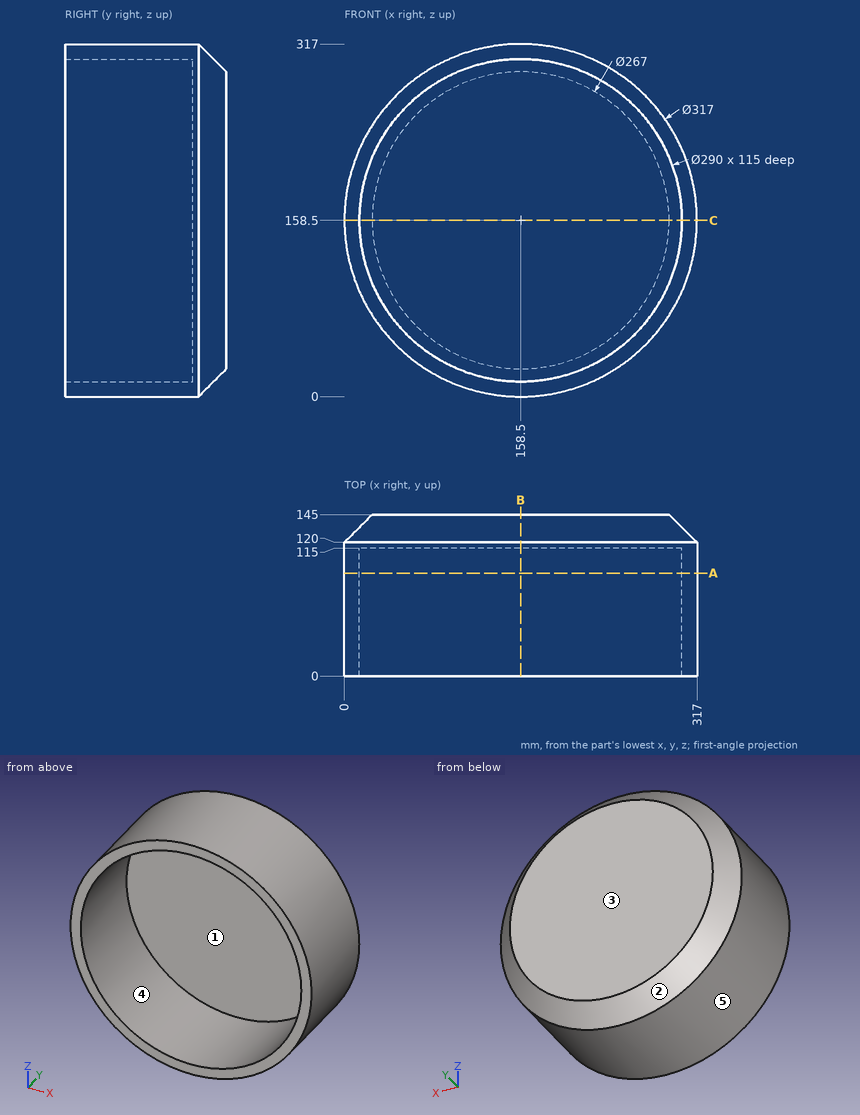
Here's the drawing with two shaded views (mm, measured from the low corner). I have some questions. A direction names the side the tool comes from. Coordinates: 2 decimals unless noted, no trailing zeros. Order: outer loops, then holes, each group sorted by start corner. A loop starts at its lowest first (then second) coordinate and runs counter-clockwise, first axis right, second up.
Q1. Thinking about a two-plate mould opening in X: for the marked faces 3, 4 and 5, which applies, released by +X, released by -X, zero draft, split by the parting line, or undercut?
Q2. Suppose I cut it at B-B on x = 158.5. Please give me the cut outline in (y, z), and give its area (3 significant figures).
Q3. Suppose I cut it at A-A on y = 92.5. Please give me the cut outline in (x, z), and give its area (3 significant figures).
Q4. Suppose I cut it at C-C on z = 158.5. Please give me the cut outline in (x, y), and give its area (3 significant figures).
Q5. Will these pins go through, and if not, where does the flat tip stop? pin 1 (12 mm diameter, centred on x = 252, y = 27.5, fed in from +Z); pin 2 (4 mm diameter, centred on y = 122, z = 66.5, fed in from -X); pin 3 (3 mm diameter, centred on x = 76.5, y = 107, fed in from -Z).
Q6. Which directions (+Z, -Z, +X, -X, +Y, -Y) give clear straight access to the entire face, cutting with the end or side of a thin tool? Please do the marked faces 1 and 2.
Q7. Please list where these lines run through material, in increasing order: L1, parallel to Z at x = 158, y = 70; L2, parallel to Y at x = 218, z = 103.
Answer:
1. face 3: zero draft
1. face 4: undercut
1. face 5: split by the parting line
2. outline: (0, 0) - (120, 0) - (145, 25) - (145, 292) - (120, 317) - (0, 317) - (0, 303.5) - (115, 303.5) - (115, 13.5) - (0, 13.5) - close
2. area: 12,000 mm2
3. outline: circle Ø317 at (158.5, 158.5); hole circle Ø290 at (158.5, 158.5)
3. area: 12,900 mm2
4. outline: (0, 0) - (13.5, 0) - (13.5, 115) - (303.5, 115) - (303.5, 0) - (317, 0) - (317, 120) - (292, 145) - (25, 145) - (0, 120) - close
4. area: 12,000 mm2
5. pin 1: stops at z = 290.66
5. pin 2: stops at x = 29.05
5. pin 3: stops at z = 21.96
6. face 1: -Y
6. face 2: +Y
7. L1: z = 0 to 13.5, 303.5 to 317
7. L2: y = 115 to 145
